Part model, mm, in its own coordinate system. A direction names the side the tool comes from. Give positions to 0.01 mm unless a question says otherwise; leave off trailing zeros. Write each loop counter-clockwise with the first axis right and the second up, starting at its lowest first coordinate (ties: lowest second). Pieces come first, ordered by that corner, then holes. Notation, with made-up numbers: M 17.25,20.25 L 49.25,20.25 A29 cw 49.25,50.25 Z; hole C -25.5,20 d11. An arc over 180 degrees is marked long. Answer as CSV lines item,"result". Start each with the question number.
1) Pin check, flat tips, straight feed: pin 1 Ø2 at (x, y) = (5.5, 133.5) entering from -Z; pin 2 Ø4 at (y, z) = (224.5, -0.5) entering from -X; pin 3 Ø1 at (x, z) = (-1, 22.5) entering from +Y. Stop position of each tip, or through.
2) Slice it at B-B, the plane y = 301.5. Give the cut face in (x, z), plus the area to 3 significant figures.
3) Slice it at D-D, the plane y = 49. Give the cut face in (x, z).
4) Slice it at C-C, the plane z = -6. Give the cut face in (x, y), plus the area to 3 significant figures.
5) Wall check: line 1 along Y through (x, z) = (-1, 24); line 2 along Y through (x, z) = (11, 18); line 3 along Z through (x, y) = (7, 321). Give the ranges that are in metal, low to high. Write a range as from..to.
6) Mould opens along Y. For faces 4 (the flat face through (0, 342.9, 35)), 5 (the flat face through (0, 317, 31.75)), 6 (the flat face through (0, 311, -38.1)) say: pulls with the +Y half, pulls with the -Y half, needs draft (parallel to the pull), parting line crosses it, or undercut.
7) Slice it at A-A, the plane x = 0. Give the cut face in (y, z).
8) Tool access for faces 1 (the flat face through (-12.7, 290, 1)), 2 (the cylindrical face through (-2.75, 150.62, 12.4)), 3 (the flat face through (0, 292.1, 0)): list every direction of +Z, -Z, +X, -X, +Y, -Y with a clear straight run to the whole face (end or side of a thin tool).
```python
from build123d import *

# Parameters (mm, degrees)
SKETCH2_R           = 25.4
BOSS_EXTRUDE1_DEPTH = 25.4
SKETCH3_R           = 12.7
BOSS_EXTRUDE2_DEPTH = 254
SKETCH4_W           = 25.4
SKETCH4_H           = 76.2
BOSS_EXTRUDE3_DEPTH = 12.7
SKETCH5_W           = 25.4
SKETCH5_H           = 6.35
BOSS_EXTRUDE4_DEPTH = 50.8
SKETCH6_R           = 6.35
BOSS_EXTRUDE5_DEPTH = 69.85
SKETCH7_R           = 25.4
BOSS_EXTRUDE6_DEPTH = 25.4


with BuildPart() as part:
    # Sketch2 → Boss-Extrude1 (new body)
    with BuildSketch(Plane(origin=(0, 0, 0), x_dir=(1, 0, 0), z_dir=(0, 1, 0))):
        Circle(SKETCH2_R)
    extrude(amount=BOSS_EXTRUDE1_DEPTH)

    # Sketch3 → Boss-Extrude2 (add)
    with BuildSketch(Plane(origin=(0, 25.4, 0), x_dir=(1, 0, 0), z_dir=(0, 1, 0))):
        Circle(SKETCH3_R)
    extrude(amount=BOSS_EXTRUDE2_DEPTH)

    # Sketch4 → Boss-Extrude3 (add)
    with BuildSketch(Plane(origin=(0, 279.4, 0), x_dir=(1, 0, 0), z_dir=(0, 1, 0))):
        Rectangle(SKETCH4_W, SKETCH4_H)
    extrude(amount=BOSS_EXTRUDE3_DEPTH)

    # Sketch5 → Boss-Extrude4 (add)
    with BuildSketch(Plane(origin=(0, 292.1, 0), x_dir=(1, 0, 0), z_dir=(0, 1, 0))):
        with Locations((0, 34.925)):
            Rectangle(SKETCH5_W, SKETCH5_H)
        with Locations((0, -34.925)):
            Rectangle(SKETCH5_W, SKETCH5_H)
    extrude(amount=BOSS_EXTRUDE4_DEPTH)

    # Sketch6 → Boss-Extrude5 (add)
    with BuildSketch(Plane.XY.offset(38.1)):
        with Locations((0, 330.2)):
            Circle(SKETCH6_R)
    extrude(amount=-BOSS_EXTRUDE5_DEPTH)

    # Sketch7 → Boss-Extrude6 (add)
    with BuildSketch(Plane.XZ):
        Circle(SKETCH7_R)
    extrude(amount=BOSS_EXTRUDE6_DEPTH)


solid = part.part
```
Found:
1,pin 1,"z = -11.88"
1,pin 2,"x = -12.7"
1,pin 3,"y = 336.53"
2,outline,"M -12.7,-38.1 L 12.7,-38.1 L 12.7,-31.75 L -12.7,-31.75 Z; M -12.7,31.75 L 12.7,31.75 L 12.7,38.1 L -12.7,38.1 Z"
2,area,"323 mm²"
3,outline,"C 0,0 d25.4"
4,outline,"M -24.68,-25.4 L 24.68,-25.4 L 24.68,25.4 L 11.19,25.4 L 11.19,279.4 L 12.7,279.4 L 12.7,292.1 L -12.7,292.1 L -12.7,279.4 L -11.19,279.4 L -11.19,25.4 L -24.68,25.4 Z; C 0,330.2 d12.7"
4,area,"8,640 mm²"
5,line 1,"-25.4..25.4, 279.4..292.1, 323.93..336.47"
5,line 2,"-25.4..25.4, 279.4..292.1"
5,line 3,"-38.1..-31.75, 31.75..38.1"
6,face 4,"pulls with the +Y half"
6,face 5,"undercut"
6,face 6,"needs draft"
7,outline,"M -25.4,-25.4 L 25.4,-25.4 L 25.4,-12.7 L 279.4,-12.7 L 279.4,-38.1 L 342.9,-38.1 L 342.9,-31.75 L 336.55,-31.75 L 336.55,31.75 L 342.9,31.75 L 342.9,38.1 L 279.4,38.1 L 279.4,12.7 L 25.4,12.7 L 25.4,25.4 L -25.4,25.4 Z; hole M 292.1,-31.75 L 323.85,-31.75 L 323.85,31.75 L 292.1,31.75 Z"
8,face 1,"+Z, -Z, -X, +Y"
8,face 2,"none"
8,face 3,"+X, -X"
